Model file for the job. Use its own axes, mm. Face numbers are marked on the shaded views. Coordinates: 2 decimals unless noted, no trailing zeros. Write each loop counter-clockwise with the first axis right and the second up, starting at its lowest first coordinate (ties: lowest second). Pieces come first, ordered by that corner, then holes.
Q1. Pin check, flat tips, straight feed: P1, Ø1, axis at x = 19, y = 14, coming from the -Z side; P2, Ø1.3, axis at x = 18.5, z = -1.5, coming from the +Y side; P3, Ø2, axis at y = -19.5, z = -1.5, coming from the -X side. Stop position of each tip, or through.
Q2. Band-saw the part on A-A, the plane y = 16. Write the cut outline in (x, z), plus the area to 3 significant figures.
Q3. Band-saw the part on D-D, the plane z = -1.25. Write the cut outline in (x, y), plus the area to 3 significant figures.
Q4. Drill centre lines: probe 1 along Y at (x, z) = (0, 3); probe 2 along Z at (x, y) = (-4.5, 10). Where is each one in solid material? Low to high.
Q5. Band-saw the part on B-B, the plane x = 18. Write the cut outline in (y, z), plus the area to 3 significant figures.
Q6. Band-saw the part on C-C, the plane z = 4.5. Write the cut outline in (x, y).
Q7. Pull direction X, two halves, no side cores. Call the marked faces 1 and 2: released by +X, released by -X, zero draft, split by the parting line, or undercut.
from build123d import *

# Parameters (mm, degrees)
F0_W     = 50.8
F0_H     = 50.8
F1_DEPTH = 2.54
F2_W     = 2.54
F2_H     = 45.72
F3_DEPTH = 2.54
F4_W     = 6.35
F4_H     = 6.35
F5_DEPTH = 2.54


with BuildPart() as f1:
    # F0 (on Top) → F1 (new body)
    with BuildSketch(Plane.XY):
        Rectangle(F0_W, F0_H)
    extrude(amount=F1_DEPTH)

    # F2 (on face) → F3 (join)
    with BuildSketch(Plane.XY.offset(2.54)):
        with Locations((-24.13, 0)):
            Rectangle(F2_W, F2_H)
        Polygon((25.4, 25.4), (-25.4, 25.4), (-25.4, 22.86), (-22.86, 22.86), (22.86, 22.86), (25.4, 22.86), align=None)
        Polygon((25.4, -25.4), (25.4, 22.86), (22.86, 22.86), (22.86, -22.86), (22.86, -25.4), align=None)
        Polygon((-22.86, -22.86), (-25.4, -22.86), (-25.4, -25.4), (22.86, -25.4), (22.86, -22.86), align=None)
    extrude(amount=F3_DEPTH)

    # F4 (on face) → F5 (join)
    with BuildSketch(Plane(origin=(0, 0, 0), x_dir=(1, 0, 0), z_dir=(0, 0, -1))):
        with Locations((19.685, 19.685)):
            Rectangle(F4_W, F4_H)
    extrude(amount=F5_DEPTH)


solid = f1.part
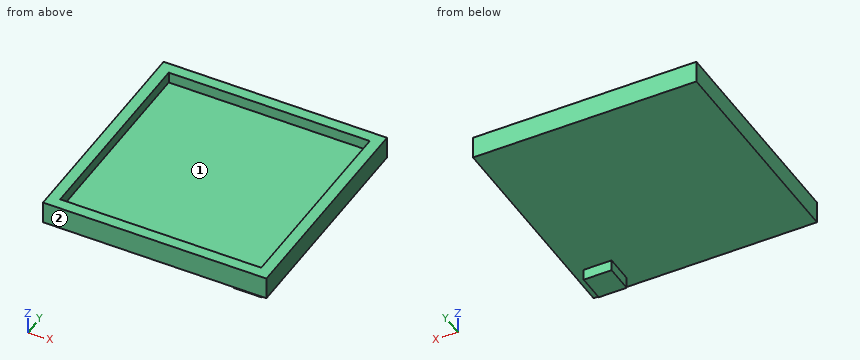
Answer sheet:
1. P1: stops at z = 0
1. P2: stops at y = -16.51
1. P3: stops at x = 16.51
2. outline: (-25.4, 0) - (25.4, 0) - (25.4, 5.08) - (22.86, 5.08) - (22.86, 2.54) - (-22.86, 2.54) - (-22.86, 5.08) - (-25.4, 5.08) - close
2. area: 142 mm2
3. outline: (16.51, -22.86) - (22.86, -22.86) - (22.86, -16.51) - (16.51, -16.51) - close
3. area: 40.3 mm2
4. probe 1: y = -25.4 to -22.86, 22.86 to 25.4
4. probe 2: z = 0 to 2.54
5. outline: (-25.4, 0) - (-22.86, 0) - (-22.86, -2.54) - (-16.51, -2.54) - (-16.51, 0) - (25.4, 0) - (25.4, 5.08) - (22.86, 5.08) - (22.86, 2.54) - (-22.86, 2.54) - (-22.86, 5.08) - (-25.4, 5.08) - close
5. area: 158 mm2
6. outline: (-25.4, -25.4) - (25.4, -25.4) - (25.4, 25.4) - (-25.4, 25.4) - close; hole (-22.86, -22.86) - (22.86, -22.86) - (22.86, 22.86) - (-22.86, 22.86) - close
7. face 1: undercut
7. face 2: zero draft
